The listing builds one solid part. Answer for the finished solid, in the listing's coordinates (mm). Face numbers are marked on the shaded views. Coordinates: 2 decimals unless noted, no trailing zeros. Loops run counter-clockwise (first coordinate to the right, second up) from the corner with the lowest first, then second, coordinate; pieces in that order, holes last. Notation, with made-up numbers: M -15.75,-14 L 35.25,-14 A13 ccw 35.25,-3 Z; hole C 58,-1 d2. An arc over 180 degrees is marked long. Answer in a Markdown table with one row per item. Add a question column.
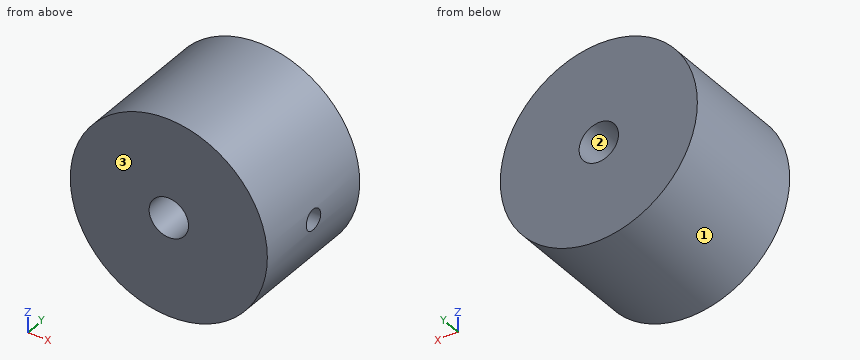
Autodesk Inventor part; units mm, degrees
ref_plane "XZ Plane" through (0, 0, 0) normal (0, 1, 0) x (-1, 0, 0)
ref_plane "XY Plane" through (0, 0, 0) normal (0, 0, 1) x (1, 0, 0)
sketch "草图1" plane through (0, 0, 0) normal (0, 1, 0) x (-1, 0, 0)
  circle A0 centre (0, 0) radius 7.5
  dimension "d0" = 15
extrude "拉伸1" add sketch "草图1" along normal blind 10
sketch "草图2" plane through (0, 10, 0) normal (0, 1, 0) x (1, 0, 0)
  circle A0 centre (0, 0) radius 1.5
  circle A1 centre (0, 0) radius 7.5
  dimension "d3" = 3
  dimension "d4" = 0
  dimension "d5" = 0
extrude "拉伸2" cut sketch "草图2" against normal blind 10 contours A0
sketch "草图3" plane through (0, 0, 0) normal (0, -1, 0) x (1, 0, 0)
  point P0 (0, 0)
ref_plane "工作平面1" through (7.5, 0, 0) normal (1, 0, 0) x (0, 1, 0)
sketch "草图4" plane through (7.5, 0, 0) normal (1, 0, 0) x (0, 1, 0)
  line L0 (0, -7.5) -> (0, 7.5)
  line L1 (10, -7.5) -> (10, 7.5)
  line L2 (0, 7.5) -> (10, 7.5)
  line L3 (0, -7.5) -> (10, -7.5)
  point P0 (0, 0)
sketch "草图5" plane through (7.5, 0, 0) normal (1, 0, 0) x (0, 1, 0)
  line L0 (10, -7.5) -> (10, 7.5)
  point P0 (0, 0)
  point P1 (5, 0)
  dimension "d8" = 5
hole "孔1" at (7.5, 5, 0) direction (-1, 0, 0) diameter 1.567 depth 3 tip angle 118
properties part number "微型联轴器"
(1) Each of these flat-tipped pins is pushed along its axis until it touches: pin 1 (1 mm diameter, centred on x = -4, y = 3, fed in from +Z); pin 2 (3 mm diameter, centred on x = 3, y = 7, fed in from -Z). Where does it stop, or does it pass through?
(2) A cutting plane is placed at B-B (x = 0). Give the vertices of the cut face in (y, z).
(3) Straight lines are drawn through the part: line 1 (X direction, y = 4, z = 0); line 2 (Y direction, x = 5.2, z = 0). For each, find the intervals that lie inside material, in ascending order.
(4) A cutting plane is placed at D-D (x = 5.25). Give the vertices of the cut face in (y, z).
(5) The mould has two halves that part along X. Classify the marked faces 1, 2 and 3: released by +X, released by -X, zero draft, split by the parting line, or undercut.
(6) A cutting plane is placed at C-C (y = 6.5). Give the vertices of the cut face in (x, z), plus the area to 3 significant figures.
(7) A cutting plane is placed at A-A (z = 1). Give the vertices of the cut face in (x, y).
Solved:
| question | item | result |
|---|---|---|
| 1 | pin 1 | stops at z = 6.63 |
| 1 | pin 2 | stops at z = -7.35 |
| 2 | outline | M 0,-7.5 L 10,-7.5 L 10,-1.5 L 0,-1.5 Z; M 0,1.5 L 10,1.5 L 10,7.5 L 0,7.5 Z |
| 3 | line 1 | x = -7.5 to -1.5, 1.5 to 7.5 |
| 3 | line 2 | y = 0 to 4.22, 5.78 to 10 |
| 4 | outline | M 0,-5.36 L 10,-5.36 L 10,5.36 L 0,5.36 Z; hole C 5,0 d1.57 |
| 5 | face 1 | split by the parting line |
| 5 | face 2 | undercut |
| 5 | face 3 | zero draft |
| 6 | outline | C 0,0 d15; hole C 0,0 d3 |
| 6 | area | 170 mm² |
| 7 | outline | M -7.43,0 L -1.12,0 L -1.12,10 L -7.43,10 Z; M 1.12,0 L 7.43,0 L 7.43,10 L 1.12,10 Z |
